Autodesk Inventor part; units mm, degrees
ref_plane "YZ Plane" through (0, 0, 0) normal (1, 0, 0) x (0, 1, 0)
ref_plane "XZ Plane" through (0, 0, 0) normal (0, 1, 0) x (-1, 0, 0)
ref_plane "XY Plane" through (0, 0, 0) normal (0, 0, 1) x (1, 0, 0)
sketch "Sketch1" plane through (0, 0, 0) normal (0, 0, 1) x (1, 0, 0)
  line L0 (0, 0) -> (44.45, 0)
  line L1 (44.45, 0) -> (44.45, 46.99)
  line L2 (44.45, 46.99) -> (0, 46.99)
  line L3 (0, 46.99) -> (0, 0)
  dimension "d0" = 46.99
  dimension "d1" = 44.45
revolve "Revolution1" add sketch "Sketch1" angle 360 about axis through (0, 0, 0) along (1, 0, 0)
chamfer "Chamfer1" distance 3.175 angle 45 2 edges at (44.45, -46.99, 0) (0, -46.99, 0)
sketch "Sketch2" plane through (44.45, 0, 0) normal (1, 0, 0) x (0, 0, -1)
  circle A0 centre (0, 0) radius 43.815
  line L0 (6.4158, 0) -> (3.2079, -5.5562)
  line L1 (3.2079, -5.5562) -> (-3.2079, -5.5562)
  line L2 (-3.2079, -5.5562) -> (-6.4158, 0)
  line L3 (-6.4158, 0) -> (-3.2079, 5.5563)
  line L4 (-3.2079, 5.5563) -> (3.2079, 5.5563)
  line L5 (3.2079, 5.5563) -> (6.4158, 0)
  dimension "d6" = 11.1125
extrude "Extrusion1" cut sketch "Sketch2" against normal through all contours L0 L1 L2 L3 L4 L5
properties part number "Wheel Temp"
Read the model definition and answer for the solid it produces. Units are mm, in the model's axes. A direction names the side the tool comes from. Give positions to 0.01 mm unless a question says otherwise; leave off trailing zeros. Write each loop counter-clockwise with the first axis right and the second up, starting at its lowest first coordinate (ties: lowest second). Pieces come first, ordered by that corner, then holes. Notation, with made-up numbers: (10.5, -29.5) -> (43.5, -29.5) arc R18 ccw to (43.5, -11.5) -> close; hole circle Ø8 at (-23, 35). An arc over 180 degrees is marked (long way). Answer in a Markdown table with one row per item.
1) Determine the mould class of faces 1 (the flat face through (22.536, -2.739, -4.834)), 2 (the conical face through (44.25, -9.54, 42.97)), 3 (the flat face through (44.45, -1, -9)) for opening direction Z: released by +Z, released by -Z, zero draft, split by the parting line, or undercut.
Results list:
| item | result |
|---|---|
| face 1 | undercut |
| face 2 | split by the parting line |
| face 3 | zero draft |
2) Each of these flat-tipped pins is pushed along its axis until it touches: pin 1 Ø10 at (x, y) = (8, 12.5) entering from +Z; pin 2 Ø5 at (x, z) = (24, 30.5) entering from +Y; pin 3 Ø1 at (x, z) = (27, -30) entering from -Y. Where does it stop, or does it pass through?
Results list:
| item | result |
|---|---|
| pin 1 | z = 46.39 |
| pin 2 | y = 37.74 |
| pin 3 | y = -36.58 |
3) Section A-A on z = 0 is taken. Give the vertices of the cut face in (x, y) (3 decimals), plus the area to 3 significant figures.
Results list:
| item | result |
|---|---|
| outline | (0, -43.815) -> (3.175, -46.99) -> (41.275, -46.99) -> (44.45, -43.815) -> (44.45, -5.556) -> (0, -5.556) -> close; (0, 5.556) -> (44.45, 5.556) -> (44.45, 43.815) -> (41.275, 46.99) -> (3.175, 46.99) -> (0, 43.815) -> close |
| area | 3,660 mm^2 |
4) Section B-B on x = 13 is taken. Give the vertices of the cut face in (y, z).
Results list:
| item | result |
|---|---|
| outline | circle Ø93.98 at (0, 0); hole (-5.56, -3.21) -> (0, -6.42) -> (5.56, -3.21) -> (5.56, 3.21) -> (0, 6.42) -> (-5.56, 3.21) -> close |
5) A tool of negligible diameter and unlimited length cuts with its end or side. For faces 4 (the flat face through (23, -5.556, 0)), 5 (the flat face through (0, -1, -9)), from which of +Z, -Z, +X, -X, +Y, -Y can it reach the whole face along a straight path? Write none if from no direction.
Results list:
| item | result |
|---|---|
| face 4 | +X, -X |
| face 5 | +Z, -Z, -X, +Y, -Y |
6) Straight lines are drawn through the part: line 1 (Y direction, x = 28.5, z = -0.5); line 2 (Z direction, x = 23, y = 17); line 3 (Z direction, x = 17, y = 6). For each, find the intervals that lie inside material, in ascending order. Write a range as [from, to].
Results list:
| item | result |
|---|---|
| line 1 | [-46.99, -5.56], [5.56, 46.99] |
| line 2 | [-43.81, 43.81] |
| line 3 | [-46.61, 46.61] |
